```python
from build123d import *

# Parameters (mm, degrees)
F0_R     = 7
F1_DEPTH = 10
F2_R     = 2.5
F3_DEPTH = 39.001
F4_R     = 2.5
F5_R     = 1.25
F6_DEPTH = 3


with BuildPart() as f1:
    # F0 (on Front) → F1 (new body, symmetric)
    with BuildSketch(Plane.XZ):
        with BuildLine():
            ThreePointArc((-1.5, -15.9295323221), (0, 16), (1.5, -15.9295323221))
            Line((1.5, -15.9295323221), (1.5, -34.9295323221))
            Line((1.5, -34.9295323221), (15, -34.9295323221))
            Line((15, -34.9295323221), (15, -18.7349939952))
            ThreePointArc((15, -18.7349939952), (20.9400506806, -11.7266481782), (23.8117617996, -3))
            Line((23.8117617996, -3), (42.3508893593, -3))
            ThreePointArc((42.3508893593, -3), (65.1980390272, -8.0622577483), (55, 13))
            ThreePointArc((55, 13), (46.9377422517, 10.1980390272), (42.3508893593, 3))
            Line((42.3508893593, 3), (23.8117617996, 3))
            ThreePointArc((23.8117617996, 3), (22.5542038346, 8.2041385525), (20.1742410018, 13))
            ThreePointArc((20.1742410018, 13), (-16.0770225308, 17.8193531461), (-15, -18.7349939952))
            Line((-15, -18.7349939952), (-15, -34.9295323221))
            Line((-15, -34.9295323221), (-1.5, -34.9295323221))
            Line((-1.5, -34.9295323221), (-1.5, -15.9295323221))
        make_face()
        with Locations((55, 0)):
            Circle(F0_R, mode=Mode.SUBTRACT)
    extrude(amount=F1_DEPTH, both=True)

    # F2 (on face) → F3 (cut, through all)
    with BuildSketch(Plane.YZ.offset(15)):
        with Locations((0, -27.9295323221)):
            Circle(F2_R)
    extrude(amount=-F3_DEPTH, mode=Mode.SUBTRACT)

    # F4
    f4_edges = [f1.edges().sort_by_distance(p)[0] for p in [
        (23.811762, 5, 3),
        (23.811762, -5, 3),
        (23.811762, 5, -3),
        (23.811762, -5, -3),
    ]]
    fillet(f4_edges, radius=F4_R)

    # F5
    f5_edges = [f1.edges().sort_by_distance(p)[0] for p in [
        (42.350889, 5, -3),
        (42.350889, -5, -3),
        (42.350889, 5, 3),
        (42.350889, -5, 3),
    ]]
    fillet(f5_edges, radius=F5_R)

    # F0 (on Front) → F6 (join, symmetric)
    with BuildSketch(Plane.XZ):
        with BuildLine():
            Line((55, 13), (20.1742410018, 13))
            ThreePointArc((20.1742410018, 13), (22.5542038346, 8.2041385525), (23.8117617996, 3))
            Line((23.8117617996, 3), (42.3508893593, 3))
            ThreePointArc((42.3508893593, 3), (46.9377422517, 10.1980390272), (55, 13))
        make_face()
    extrude(amount=F6_DEPTH, both=True)


solid = f1.part
```
Can you work these out from the model? Positions are in its coordinate system, mm. A direction names the side the tool comes from. Round coordinates to 2 decimals unless told otherwise and drop trailing zeros. Loops run counter-clockwise (first coordinate to the right, second up) from the corner with the lowest first, then second, coordinate; pieces in that order, holes last. Notation, with made-up numbers: M 46.25,-22.75 L 66.25,-22.75 A10 ccw 66.25,-15.75 Z; hole C -1.75,14 d10. An arc over 180 degrees is marked long. Answer as a JSON object with one key per item and string values. Group by question number.
Q1. Imagine slicing it at B-B, the plane z = 0. Please give me the cut outline in (x, y).
Q2. Imagine slicing it at C-C, the plane y = 7. Please give me the cut outline in (x, z) (3 decimals).
Q3. Please list where these lines run through material, in increasing order: L1, parallel to X at y = 4.75, z = -24; L2, parallel to Z at x = -7.75, y = 0; L3, parallel to Z at x = 8.5, y = 0.
Q4. We'd pull the mould along X, two halves only. Please class faces 6 (the flat face through (15, 0, -25)), 7 (the flat face through (-1.5, 0, -23)), 8 (the flat face through (15, -10, -10)), 9 (the flat face through (-15, 0, -25)): +X half, -X half, draft (parallel to the pull), parting line (faces both ways), or undercut.
Q5. Imagine slicing it at D-D, the plane z = -24.5. Please give me the cut outline in (x, y), then the cut area to 3 significant figures.
Q6. Will these pins go through, and if not, where does the flat tip stop? pin 1 (3 mm diameter, centred on x = 31, y = 1, fed in from +Z); pin 2 (6 mm diameter, centred on y = 0, z = -27.93, fed in from +X); pin 3 (6.5 mm diameter, centred on y = 0, z = -27.93, fed in from -X).
Q7. Imagine slicing it at A-A, the plane y = 0. Please give me the cut outline in (x, z) (3 decimals).
Q8. On a 3-axis mill with a long thin cutter (end or side, diameter ignored), from which of +Z, -Z, +X, -X, +Y, -Y can I reach the whole of each face in a straight line? I mean faces 1 (the cylindrical face through (24.3, 6.5, 3.6)), 2 (the flat face through (34, -7, 3)), 3 (the flat face through (8, 0, -34.93)), 4 (the flat face through (38, 0, 13)), 5 (the flat face through (1.5, 0, -25)). Say none if no direction works.
Findings:
{
 "1": {"outline": "M -24,-10 L -16,-10 L -16,10 L -24,10 Z; M 16,-10 L 48,-10 L 48,10 L 16,10 Z; M 62,-10 L 68,-10 L 68,10 L 62,10 Z"},
 "2": {"outline": "M -15,-34.93 L -1.5,-34.93 L -1.5,-15.93 A16 cw long 1.5,-15.93 L 1.5,-34.93 L 15,-34.93 L 15,-18.735 A24 ccw 23.477,-4.981 A2.5 cw 25.923,-3 L 41.399,-3 A1.25 cw 42.592,-3.877 A13 ccw long 42.592,3.877 A1.25 cw 41.399,3 L 25.923,3 A2.5 cw 23.477,4.981 A24 ccw long -15,-18.735 Z; hole C 55,0 d14"},
 "3": {"L1": "x = -15 to -1.5, 1.5 to 15", "L2": "z = -34.93 to -30.43, -25.43 to -14, 14 to 22.71", "L3": "z = -34.93 to -30.43, -25.43 to -13.56, 13.56 to 22.44"},
 "4": {"face 6": "+X half", "face 7": "undercut", "face 8": "draft", "face 9": "-X half"},
 "5": {"outline": "M -15,-10 L -1.5,-10 L -1.5,10 L -15,10 Z; M 1.5,-10 L 15,-10 L 15,10 L 1.5,10 Z", "area": "540 mm2"},
 "6": {"pin 1": "stops at z = 13", "pin 2": "stops at x = 15", "pin 3": "stops at x = -15"},
 "7": {"outline": "M -15,-34.93 L -1.5,-34.93 L -1.5,-30.43 L -15,-30.43 Z; M -15,-25.43 L -1.5,-25.43 L -1.5,-15.93 A16 cw long 1.5,-15.93 L 1.5,-25.43 L 15,-25.43 L 15,-18.735 A24 ccw 23.477,-4.981 A2.5 cw 25.923,-3 L 41.399,-3 A1.25 cw 42.592,-3.877 A13 ccw long 55,13 L 20.174,13 A24 ccw long -15,-18.735 Z; M 1.5,-34.93 L 15,-34.93 L 15,-30.43 L 1.5,-30.43 Z; hole C 55,0 d14"},
 "8": {"face 1": "+Z, +Y", "face 2": "+Z, -Y", "face 3": "-Z, +X, -X, +Y, -Y", "face 4": "+Z, +X, +Y, -Y", "face 5": "-Z, +Y, -Y"}
}
